Autodesk Inventor part; units mm, degrees
ref_plane "Work Plane1" through (0, 300, 0) normal (0, 1, 0) x (1, 0, 0)
ref_plane "YZ Plane" through (0, 0, 0) normal (1, 0, 0) x (0, 1, 0)
ref_plane "XZ Plane" through (0, 0, 0) normal (0, 1, 0) x (-1, 0, 0)
sketch "Sketch1" plane through (0, 0, 0) normal (0, 1, 0) x (-1, 0, 0)
  line L0 (-5, -5) -> (5, -5)
  line L1 (5, -5) -> (5, 5)
  line L2 (5, 5) -> (-5, 5)
  line L3 (-5, 5) -> (-5, -5)
  line L4 (-5, -5) -> (5, 5) construction
  line L5 (5, -5) -> (-5, 5) construction
  line L6 (-4, -4) -> (4, -4)
  line L7 (4, -4) -> (4, 4)
  line L8 (4, 4) -> (-4, 4)
  line L9 (-4, 4) -> (-4, -4)
  line L10 (-4, -4) -> (4, 4) construction
  line L11 (4, -4) -> (-4, 4) construction
  point P0 (0, 0)
  dimension "d0" = 10
  dimension "d1" = 10
  dimension "d2" = 8
  dimension "d3" = 8
extrude "Extrusion1" add sketch "Sketch1" along normal blind 600
sketch "Sketch2" plane through (5, 0, -5) normal (1, 0, 0) x (0, 0, -1)
  line L0 (-10, 600) -> (0, 600)
  line L1 (-10, 0) -> (0, 0)
  point P0 (-5, 0)
  point P1 (-5, 545)
  point P2 (-5, 525)
  point P3 (-5, 590)
  point P4 (-5, 555)
  point P5 (-5, 575)
  point P6 (-5, 10)
  point P7 (-5, 25)
  point P8 (-5, 35)
  point P9 (-5, 55)
  point P10 (-5, 107.8006)
  dimension "d6" = 55
  dimension "d7" = 20
  dimension "d21" = 10
  dimension "d23" = 35
  dimension "d24" = 15
  dimension "d25" = 10
  dimension "d26" = 15
  dimension "d27" = 10
  dimension "d28" = 20
hole "Hole1" at (5, 545, 0) at (5, 525, 0) at (5, 590, 0) at (5, 555, 0) at (5, 575, 0) at (5, 10, 0) at (5, 25, 0) at (5, 35, 0) at (5, 55, 0) direction (-1, 0, 0) diameter 3 depth 80.45
sketch "Sketch3" plane through (-5, 0, -5) normal (0, 0, -1) x (-1, 0, 0)
  line L0 (-10, 600) -> (0, 600)
  circle A0 centre (-5, 595) radius 1.5
  line L1 (-10, 0) -> (0, 0)
  circle A1 centre (-5, 5) radius 1.75
  point P0 (-5, 0)
  dimension "d15" = 5
  dimension "d16" = 3
  dimension "d19" = 5
  dimension "d20" = 3.5
extrude "Extrusion2" cut sketch "Sketch3" against normal blind 600
ref_plane "Work Plane1" through (0, 300, 0) normal (0, 1, 0) x (1, 0, 0)
properties part number "10x10x600" material "アルミニウム 6061"
Could you check a few things on this model? Use its own coordinates, in mm. Give positions to 0.01 mm unless a question says otherwise; leave off trailing zeros. Write each loop counter-clockwise with the first axis right and the second up, starting at its lowest first coordinate (ties: lowest second). Pieces come first, ordered by that corner, then holes. Notation, with made-up numbers: (56.25, 8) - (67.25, 8) arc R16 ccw to (67.25, 20) - close; hole circle Ø8 at (75, -30). An arc over 180 degrees is marked (long way). Use CSV: the item, a comma, the result in double quotes. Start each with the question number.
Item 1: I want a section at A-A, the plane y = 200. Please give me the cut outline in (x, z), then the cut area to 3 significant figures.
Item 2: If we mould it in two halves opening along Z, with no side actions, what happens to faces 1 (the face through (0, 296, 5)), 2 (the face through (0, 296, -5)), 3 (the face through (-5, 296, 0))? For each: pulls with the +Z half, pulls with the -Z half, needs draft (parallel to the pull), parting line crosses it, or undercut.
Item 3: I want a section at B-B, the plane x = 0. Please give me the cut outline in (y, z), then the cut area to 3 significant figures.
Item 4: I want a section at C-C, the plane z = 0. Give the number of separate pieces and of enclosed holes in the cut face, then the cut area to 3 significant figures.
Item 5: If I drill on line 1 along Y through (x, z) = (0, 4.6); line 2 along X through (y, z) = (178, -1), over which ranges is the centre line in solid material (lowest first)?
Item 6: I'm going to push a flat-ended pin straight in: pin 1 (2.5 mm diameter, centred on y = 25, z = 0, fed in from +X) (3 decimals). Where does the tip first touch, or does it pass through?
Findings:
1,outline,"(-5, -5) - (5, -5) - (5, 5) - (-5, 5) - close; hole (-4, -4) - (4, -4) - (4, 4) - (-4, 4) - close"
1,area,"36.0 mm2"
2,face 1,"pulls with the +Z half"
2,face 2,"pulls with the -Z half"
2,face 3,"needs draft"
3,outline,"(0, -5) - (3.25, -5) - (3.25, -4) - (0, -4) - close; (0, 4) - (3.25, 4) - (3.25, 5) - (0, 5) - close; (6.75, -5) - (593.5, -5) - (593.5, -4) - (6.75, -4) - close; (6.75, 4) - (593.5, 4) - (593.5, 5) - (6.75, 5) - close; (596.5, -5) - (600, -5) - (600, -4) - (596.5, -4) - close; (596.5, 4) - (600, 4) - (600, 5) - (596.5, 5) - close"
3,area,"1,190 mm2"
4,separate pieces,"20"
4,enclosed holes,"0"
4,area,"1,150 mm2"
5,line 1,"y = 0 to 3.25, 6.75 to 593.5, 596.5 to 600"
5,line 2,"x = -5 to -4, 4 to 5"
6,pin 1,"passes through"
